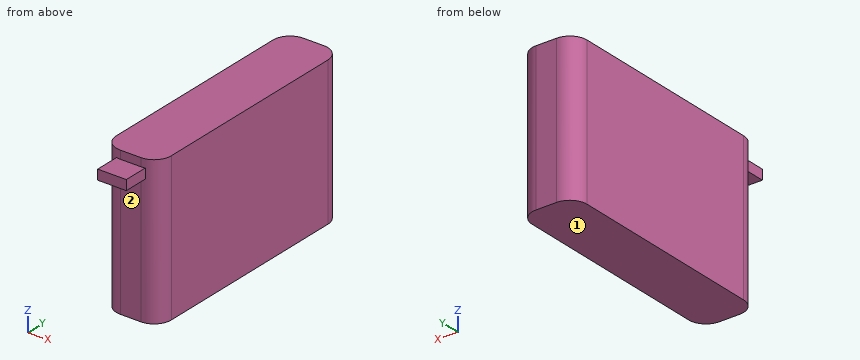
```python
from build123d import *

# Parameters (mm, degrees)
RESSALTO_EXTRUS_O4_DEPTH      = 43
RESSALTO_EXTRUS_O5_DEPTH      = 7
RESSALTO_EXTRUS_O5_DEPTH_BACK = 10
ESBO_O5_W                     = 8.350993052
ESBO_O5_H                     = 2.899650365


with BuildPart() as part:
    # Esboço4 → Ressalto-extrusão4 (new body)
    with BuildSketch(Plane.XY):
        with BuildLine():
            Line((-3, 34.5), (3, 34.5))
            ThreePointArc((3, 34.5), (6.535533906, 33.035533906), (8, 29.5))
            Line((8, 29.5), (8, -29.5))
            ThreePointArc((8, -29.5), (6.535533906, -33.035533906), (3, -34.5))
            Line((3, -34.5), (-3, -34.5))
            ThreePointArc((-3, -34.5), (-6.535533906, -33.035533906), (-8, -29.5))
            Line((-8, -29.5), (-8, 29.5))
            ThreePointArc((-8, 29.5), (-6.535533906, 33.035533906), (-3, 34.5))
        make_face()
    extrude(amount=RESSALTO_EXTRUS_O4_DEPTH)

    # Esboço5 → Ressalto-extrusão5 (add, two sides: drawn at the far end of the back side and taken through both)
    with BuildSketch(Plane.XZ.offset(34.5).offset(-RESSALTO_EXTRUS_O5_DEPTH_BACK)):
        with Locations((0, 39.158870724)):
            Rectangle(ESBO_O5_W, ESBO_O5_H)
    extrude(amount=RESSALTO_EXTRUS_O5_DEPTH + RESSALTO_EXTRUS_O5_DEPTH_BACK)


solid = part.part
```
CAD build for the part. Positions are in the model's coordinates, mm. Face numbers are marked on the shaded views. A direction names the side the tool comes from. Round coordinates to 2 decimals unless told otherwise and drop trailing zeros. Order: outer loops, then holes, each group sorted by start corner. A loop starts at its lowest first (then second) coordinate and runs counter-clockwise, first axis right, second up.
Item 1: Tool access for the marked faces 1 and 2: list every direction of +Z, -Z, +X, -X, +Y, -Y with a clear straight run to the whole face (end or side of a thin tool).
Item 2: Saw through at D-D on z = 39. Write the cut outline in (x, y), then the cut area to 3 significant figures.
Item 3: Saw through at A-A on z = 27. Write the cut outline in (x, y), then the cut area to 3 significant figures.
Item 4: Probe line 1 along Y through (x, z) = (-2.75, 17); line 2 along Y through (x, z) = (-7, 17.5); line 3 along X through (y, z) = (-30, 17). List the from-to ranges inside material, lowest first.
Item 5: Saw through at B-B on x = -0.75. Write the cut outline in (y, z).
Item 6: Pin check, flat tips, straight feed: pin 1 (3 mm diameter, centred on y = -37, z = 40, fed in from -X); pin 2 (5.5 mm diameter, centred on x = 1.5, y = -38, fed in from +Z); pin 3 (1.4 mm diameter, centred on y = -39.5, z = 39, fed in from +X). Stop position of each tip, or through.
Item 7: Saw through at C-C on y = -36. Write the cut outline in (x, z), then the cut area to 3 significant figures.
Reported:
1. face 1: -Z, +X, -X, +Y, -Y
1. face 2: -Z, +X, -X, -Y
2. outline: (-8, -29.5) arc R5 ccw to (-4.18, -34.36) - (-4.18, -41.5) - (4.18, -41.5) - (4.18, -34.36) arc R5 ccw to (8, -29.5) - (8, 29.5) arc R5 ccw to (3, 34.5) - (-3, 34.5) arc R5 ccw to (-8, 29.5) - close
2. area: 1,140 mm2
3. outline: (-8, -29.5) arc R5 ccw to (-3, -34.5) - (3, -34.5) arc R5 ccw to (8, -29.5) - (8, 29.5) arc R5 ccw to (3, 34.5) - (-3, 34.5) arc R5 ccw to (-8, 29.5) - close
3. area: 1,080 mm2
4. line 1: y = -34.5 to 34.5
4. line 2: y = -32.5 to 32.5
4. line 3: x = -7.97 to 7.97
5. outline: (-41.5, 37.71) - (-34.5, 37.71) - (-34.5, 0) - (34.5, 0) - (34.5, 43) - (-34.5, 43) - (-34.5, 40.61) - (-41.5, 40.61) - close
6. pin 1: stops at x = -4.18
6. pin 2: stops at z = 40.61
6. pin 3: stops at x = 4.18
7. outline: (-4.18, 37.71) - (4.18, 37.71) - (4.18, 40.61) - (-4.18, 40.61) - close
7. area: 24.2 mm2
